Here's how the part is built. I have some questions about the finished solid (model axes, mm). Coordinates: 2 decimals unless noted, no trailing zeros. Write each loop counter-clockwise with the first axis right and the second up, starting at its lowest first coordinate (ties: lowest second). Pieces come first, ordered by that corner, then holes.
Autodesk Inventor part; units mm, degrees
ref_plane "YZ Plane" through (0, 0, 0) normal (1, 0, 0) x (0, 1, 0)
ref_plane "XZ Plane" through (0, 0, 0) normal (0, 1, 0) x (-1, 0, 0)
ref_plane "XY Plane" through (0, 0, 0) normal (0, 0, 1) x (1, 0, 0)
sketch "Sketch1" plane through (0, 0, 0) normal (0, 0, 1) x (1, 0, 0)
  line L0 (133.35, 0) -> (428.625, 0)
  line L1 (428.625, 0) -> (428.625, 431.8)
  line L2 (428.625, 431.8) -> (0, 431.8)
  circle A0 centre (200.025, 228.6) radius 14.2875
  circle A1 centre (200.025, 228.6) radius 250.0376 construction
  circle A2 centre (376.8283, 51.7967) radius 14.2875
  line L3 (200.025, 228.6) -> (428.625, 0) construction
  line L4 (0, 152.4) -> (60.325, 152.4)
  line L5 (133.35, 79.375) -> (133.35, 0)
  arc A3 (133.35, 79.375) -> (60.325, 152.4) centre (60.325, 79.375) ccw
  line L6 (0, 431.8) -> (0, 152.4)
  point P0 (0, 0)
  dimension "d5" = 500.0752
  dimension "d0" = 428.625
  dimension "d1" = 431.8
  dimension "d2" = 28.575
  dimension "d3" = 228.6
  dimension "d4" = 228.6
  dimension "d6" = 28.575
  dimension "d7" = 152.4
  dimension "d8" = 295.275
  dimension "d9" = 73.025
extrude "Extrusion1" add sketch "Sketch1" along normal blind 3.175
sketch "Sketch2" plane through (0, 0, 3.175) normal (0, 0, 1) x (1, 0, 0)
  circle A0 centre (415.925, 12.7) radius 3.5687
  line L0 (133.35, 0) -> (428.625, 0)
  line L1 (428.625, 0) -> (428.625, 431.8)
  circle A1 centre (415.925, 76.2) radius 3.5687
  circle A2 centre (415.925, 139.7) radius 3.5687
  circle A3 centre (415.925, 203.2) radius 3.5687
  circle A4 centre (415.925, 266.7) radius 3.5687
  circle A5 centre (352.425, 12.7) radius 3.5687
  circle A6 centre (288.925, 12.7) radius 3.5687
  circle A7 centre (225.425, 12.7) radius 3.5687
  circle A8 centre (161.925, 12.7) radius 3.5687
  point P0 (0, 0)
  dimension "d12" = 7.1374
  dimension "d13" = 12.7
  dimension "d14" = 12.7
  dimension "d17" = 63.5
  dimension "d27" = 63.5
extrude "Extrusion2" cut sketch "Sketch2" against normal blind 3.175
properties part number "1073-2017 Shooter Outside Plate Left"
1) Imagine slicing it at B-B on x = 369. Please give me the cut outline in (y, z) (3 decimals).
Values follow:
outline: (0, 0) - (39.845, 0) - (39.845, 3.175) - (0, 3.175) - close; (63.749, 0) - (431.8, 0) - (431.8, 3.175) - (63.749, 3.175) - close
2) Will these pins go through, and if not, where does the flat tip stop? pin 1 (6.5 mm diameter, centred on x = 225.425, y = 12.7, fed in from -Z); pin 2 (1.6 mm diameter, centred on y = 20.5, z = 1, fed in from -X).
Values follow:
pin 1: passes through
pin 2: stops at x = 133.35
3) We'd pull the mould along X, two halves only. Please class faces 1 (the face through (390.026, 57.269, 1.565)), 2 (the face through (211, 219, 0)), 3 (the face through (206.618, 241.275, 1.565)), 4 (the face through (111.391, 131.576, 1.565)): pulls with the +X half, pulls with the -X half, needs draft (parallel to the pull), parting line crosses it, or undercut.
Values follow:
face 1: undercut
face 2: needs draft
face 3: undercut
face 4: pulls with the -X half
4) Imagine slicing it at A-A on y = 228.6. Please give me the cut outline in (x, z) (1 decimal).
Values follow:
outline: (0, 0) - (185.7, 0) - (185.7, 3.2) - (0, 3.2) - close; (214.3, 0) - (428.6, 0) - (428.6, 3.2) - (214.3, 3.2) - close
5) I need wall thicknesses on probe 1 along Y at (x, z) = (226, 1.45); probe 2 along Y at (x, z) = (366, 1.6); probe 3 along X at (y, z) = (62.5, 1.8) (3 decimals). Which ranges of each line are inside material? Lowest first, please.
Values follow:
probe 1: y = 0 to 9.18, 16.22 to 431.8
probe 2: y = 0 to 42.48, 61.12 to 431.8
probe 3: x = 133.35 to 367.364, 386.293 to 428.625
6) Imagine slicing it at D-D on x = 35. Please give me the cut outline in (y, z) (3 decimals), then the cut area to 3 significant figures.
Values follow:
outline: (152.4, 0) - (431.8, 0) - (431.8, 3.175) - (152.4, 3.175) - close
area: 887 mm2
7) Imagine slicing it at C-C on z = 1.8. Count the separate pieces of the cut face and the enclosed holes in it, then the cut area to 3 significant figures.
Values follow:
separate pieces: 1
enclosed holes: 11
area: 164,000 mm2
